from build123d import *

# Parameters (mm, degrees)
SKETCH1_R               = 8
BOSS_EXTRUDE1_DEPTH     = 26.25
SKETCH2_R               = 6
BOSS_EXTRUDE2_DEPTH     = 21.875
SKETCH3_R               = 6
BOSS_EXTRUDE3_DEPTH     = 21.875
CUT_EXTRUDE4_DEPTH      = 22.875
CUT_EXTRUDE4_DEPTH_BACK = 49.125
SKETCH7_W               = 1
SKETCH7_H               = 0.5
SKETCH9_R               = 3.175
CUT_EXTRUDE5_DEPTH      = 71
CHAMFER1_SIZE           = 1
F_3_8_24_TAPPED_HOLE1_D = 8.4328


with BuildPart() as part:
    # Sketch1 → Boss-Extrude1 (new body)
    with BuildSketch(Plane.XY):
        Circle(SKETCH1_R)
    extrude(amount=BOSS_EXTRUDE1_DEPTH)

    # Sketch2 → Boss-Extrude2 (add)
    with BuildSketch(Plane(origin=(0, 0, 0), x_dir=(-1, 0, 0), z_dir=(0, 0, -1))):
        Circle(SKETCH2_R)
    extrude(amount=BOSS_EXTRUDE2_DEPTH)

    # Sketch3 → Boss-Extrude3 (add)
    with BuildSketch(Plane.XY.offset(26.25)):
        Circle(SKETCH3_R)
    extrude(amount=BOSS_EXTRUDE3_DEPTH)

    # Sketch5 → Cut-Extrude4 (cut, two sides)
    with BuildSketch(Plane(origin=(0, 0, 0), x_dir=(-1, 0, 0), z_dir=(0, 0, -1))) as cut_extrude4_sk:
        with BuildLine():
            Line((-6, -5.291502622), (-6, 5.291502622))
            ThreePointArc((-6, 5.291502622), (-8, 0), (-6, -5.291502622))
        make_face()
        with BuildLine():
            ThreePointArc((8, 0), (7.483314774, 2.828427125), (6, 5.291502622))
            Line((6, 5.291502622), (6, -5.291502622))
            ThreePointArc((6, -5.291502622), (7.483314774, -2.828427125), (8, 0))
        make_face()
    extrude(amount=CUT_EXTRUDE4_DEPTH, mode=Mode.SUBTRACT)
    extrude(cut_extrude4_sk.sketch, amount=-CUT_EXTRUDE4_DEPTH_BACK, mode=Mode.SUBTRACT)

    # Sketch7 → Cut-Revolve1 (revolve, cut)
    with BuildSketch(Plane(origin=(0, 0, 0), x_dir=(0, 0, -1), z_dir=(1, 0, 0))):
        with Locations((20.375, 5.75)):
            Rectangle(SKETCH7_W, SKETCH7_H)
        with Locations((-46.625, 5.75)):
            Rectangle(SKETCH7_W, SKETCH7_H)
    revolve(axis=Axis((0, 0, 48.125), (0, 0, -1)), mode=Mode.SUBTRACT)

    # Sketch8 → Cut-Revolve2 (revolve, cut)
    with BuildSketch(Plane(origin=(0, 0, 0), x_dir=(0, 0, -1), z_dir=(1, 0, 0))):
        with BuildLine():
            Line((-24.25, 8), (-20.25, 8))
            ThreePointArc((-20.25, 8), (-22.25, 6), (-24.25, 8))
        make_face()
        with BuildLine():
            Line((-6, 8), (-2, 8))
            ThreePointArc((-2, 8), (-4, 6), (-6, 8))
        make_face()
    revolve(axis=Axis((0, 0, 48.125), (0, 0, -1)), mode=Mode.SUBTRACT)

    # Sketch9 → Cut-Extrude5 (cut, through all)
    with BuildSketch(Plane.XY.offset(48.125)):
        Circle(SKETCH9_R)
    extrude(amount=-CUT_EXTRUDE5_DEPTH, mode=Mode.SUBTRACT)

    # Chamfer1
    chamfer1_edges = [part.edges().sort_by_distance(p)[0] for p in [
        (-3.175, 0, -21.875),
        (-3.175, 0, 48.125),
    ]]
    chamfer(chamfer1_edges, length=CHAMFER1_SIZE)

    # 3/8-24 Tapped Hole1 (through all)
    with Locations(Plane.ZY.offset(6)):
        with Locations((13.125, 0)):
            Hole(F_3_8_24_TAPPED_HOLE1_D / 2)


solid = part.part
Input: part model. Units: mm. Frame: model coordinates. A direction names the side the tool comes from. Coordinates: 2 decimals unless noted, no trailing zeros. Loops run counter-clockwise (first coordinate to the right, second up) from the corner with the lowest first, then second, coordinate; pieces in that order, holes last.
(1) First-contact query: pin 1 Ø5 at (x, z) = (3, 40) entering from -Y; pin 2 Ø6 at (x, y) = (0.5, -1) entering from +Z; pin 3 Ø1.5 at (x, z) = (2, 13.5) entering from -Y. Flat tips, straight axial feed; report the tip coordinate or a pass-through.
(2) Pull-direction query (Z, two-part tool) for faces 1 (the face through (0.4, 6.4, 0)), 2 (the face through (-5, -3, 46.125)), 3 (the face through (-0.69, -3.1, -5.04)); classes: released by +Z, released by -Z, zero draft, split by the parting line, or undercut.
(3) Material intervals for probe 1 along X at (y, z) = (0, 41) (3 decimals); probe 2 along Z at (x, y) = (5, 4.5), sorted ascending.
(4) Section B-B on y = -2. Count the separate pieces of the cut face and the enclosed holes in it, then the cut area to 3 significant figures.
(5) Section A-A on z = -15.5. Return the cut outline in (x, y) (3 decimals), then the cut area to 3 significant figures.
(6) Set-up query: faces 4 (the face through (-5.37, -1.19, -20.38)), 5 (the face through (5.54, -2.3, 47.62)), 6 (the face through (0.4, -6.4, 26.25)). Return all of +Z, -Z, +X, -X, +Y, -Y with unobstructed straight access to the full face (end or side cutting, diameter ignored); none if empty.
Data:
1. pin 1: stops at y = -5.98
1. pin 2: stops at z = 48.07
1. pin 3: stops at y = -7.9
2. face 1: released by -Z
2. face 2: undercut
2. face 3: zero draft
3. probe 1: x = -6 to -3.175, 3.175 to 6
3. probe 2: z = 0 to 2.46, 5.54 to 20.71, 23.79 to 26.25
4. separate pieces: 4
4. enclosed holes: 0
4. area: 406 mm2
5. outline: circle Ø12 at (0, 0); hole circle Ø6.35 at (0, 0)
5. area: 81.4 mm2
6. face 4: none
6. face 5: +Z
6. face 6: +Z, -Y
